Autodesk Inventor part; units mm, degrees
ref_plane "YZ Plane" through (0, 0, 0) normal (1, 0, 0) x (0, 1, 0)
ref_plane "XZ Plane" through (0, 0, 0) normal (0, 1, 0) x (-1, 0, 0)
ref_plane "XY Plane" through (0, 0, 0) normal (0, 0, 1) x (1, 0, 0)
sketch "Эскиз1" plane through (0, 0, 0) normal (0, 1, 0) x (-1, 0, 0)
  line L0 (7.1, -15.85) -> (-7.1, -15.85)
  line L1 (-7.1, -15.85) -> (-7.1, 15.85)
  line L2 (-7.1, 15.85) -> (7.1, 15.85)
  line L3 (7.1, 15.85) -> (7.1, -15.85)
  line L4 (7.1, -15.85) -> (-7.1, 15.85) construction
  line L5 (-7.1, -15.85) -> (7.1, 15.85) construction
  line L6 (9.1, -17.85) -> (-9.1, -17.85)
  line L7 (-9.1, -17.85) -> (-9.1, 17.85)
  line L8 (-9.1, 17.85) -> (9.1, 17.85)
  line L9 (9.1, 17.85) -> (9.1, -17.85)
  point P0 (0, 0)
  dimension "d0" = 14.2
  dimension "d1" = 31.7
  dimension "d2" = 2
extrude "Выдавливание1" add sketch "Эскиз1" along normal blind 7
sketch "Эскиз2" plane through (0, 7, 0) normal (0, 1, 0) x (1, 0, 0)
  line L0 (-9.1, 17.85) -> (-9.1, -17.85)
  line L1 (-9.1, -17.85) -> (9.1, -17.85)
  line L2 (9.1, -17.85) -> (9.1, 17.85)
  line L3 (9.1, 17.85) -> (-9.1, 17.85)
  point P0 (0, 0)
extrude "Выдавливание2" add sketch "Эскиз2" along normal blind 3
sketch "Эскиз4" plane through (9.1, 0, -17.85) normal (0, 0, -1) x (-1, 0, 0)
  line L0 (0, 0) -> (0, 10) construction
  line L1 (0, 0) -> (0, 10) construction
  line L2 (0, 0) -> (18.2, 0) construction
  line L3 (18.2, 0) -> (18.2, 10) construction
  line L4 (18.2, 0) -> (18.2, 10) construction
  line L5 (0, 0) -> (0, 10)
  line L6 (0, 0) -> (0, 10)
  line L7 (18.2, 0) -> (0, 0)
  line L8 (0, 0) -> (18.2, 0)
  line L9 (18.2, 0) -> (18.2, 10)
  line L10 (5.972, 10) -> (0, 10)
  line L11 (0, 10) -> (18.2, 10)
  line L12 (0, 0) -> (0, 10)
  line L13 (0, 10) -> (0, 7)
  line L14 (2, 0) -> (2, 7)
  line L15 (2, 7) -> (16.2, 7)
  line L16 (16.2, 7) -> (16.2, 0)
  point P0 (9.1, 0)
  point P1 (18.2, 7)
  point P2 (0, 5)
  point P3 (18.2, 5)
  point P4 (16.2, 0)
  dimension "d1" = 31.7
  dimension "d15" = 2
  dimension "d16" = 2
extrude "Выдавливание4" cut sketch "Эскиз4" against normal blind 3 contours L14 L15 L16 L7
sketch "Эскиз5" plane through (0, 10, 0) normal (0, 1, 0) x (1, 0, 0)
  line L0 (0, 0) -> (0, -28.4562) construction
  circle A0 centre (0, -22.85) radius 1.6
  circle A1 centre (0, 22.85) radius 1.6
  line L1 (-9.1, -17.85) -> (9.1, -17.85)
  line L2 (9.1, 17.85) -> (-9.1, 17.85)
  arc A2 (2.6208, 25.1698) -> (-2.6208, 25.1698) centre (0, 22.85) ccw
  arc A3 (-2.6208, -25.1698) -> (2.6208, -25.1698) centre (0, -22.85) ccw
  line L3 (9.1, 17.85) -> (7.1, 17.85)
  line L4 (9.1, 17.85) -> (2.6208, 25.1698)
  line L5 (-9.1, 17.85) -> (-2.6208, 25.1698)
  line L6 (-9.1, -17.85) -> (-2.6208, -25.1698)
  line L7 (9.1, -17.85) -> (9.1, 17.85)
  line L8 (9.1, -17.85) -> (2.6208, -25.1698)
  dimension "d32" = 3.2
  dimension "d33" = 3.2
  dimension "d34" = 5
  dimension "d35" = 5
  dimension "d36" = 7
  dimension "d37" = 7
extrude "Выдавливание5" add sketch "Эскиз5" against normal blind 3
sketch "Эскиз6" plane through (0, 7, 0) normal (0, -1, 0) x (1, 0, 0)
  circle A0 centre (0, -8.65) radius 1.5 construction
  circle A1 centre (0, -8.65) radius 1.6
  point P0 (0, 0)
  dimension "d38" = 3.2
extrude "Выдавливание6" cut sketch "Эскиз6" against normal blind 10
chamfer "Фаска1" distance 1.65 angle 45 1 edges at (-1.6, 10, -8.65)
properties part number "креп_опт" material "Полипропилен"
Model file for the job. Use its own axes, mm. A direction names the side the tool comes from. Give positions to 0.01 mm unless a question says otherwise; leave off trailing zeros. Order: outer loops, then holes, each group sorted by start corner. A loop starts at its lowest first (then second) coordinate and runs counter-clockwise, first axis right, second up.
1) Saw through at D-D, the plane x = -4.25. Write the cut outline in (y, z).
2) Saw through at C-C, the plane y = 1.25. Write the cut outline in (x, z), then the cut area to 3 significant figures.
3) Saw through at A-A, the plane z = -8.65. Write the cut outline in (x, y), then the cut area to 3 significant figures.
4) Wall check: probe 1 along Z at (x, y) = (0, 7.85); probe 2 along Z at (x, y) = (0, 9.3); probe 3 along X at (y, z) = (5.25, 2). Give the ranges that are in metal, low to high.
5) Saw through at B-B, the plane y = 7.5. Write the cut outline in (x, z), then the cut area to 3 significant figures.
6) Mould opens along Z. For faces 1 (the flat face through (5.906, 8.521, -21.459)), 2 (the cylindrical face through (-0.35, 8.52, 24.41)), 3 (the flat face through (7.1, 3, -1)) say: +Z half, -Z half, draft (parallel to the pull), parting line (faces both ways), or undercut.
7) 3-axis set-ups, long thin cutter, end or side, ignore diameter. For faces 4 (the flat face through (0, 7, 21)), 5 (the flat face through (0, 3, 15.85)), 6 (the flat face through (-9.1, 5, 0)), 7 (the flat face through (7.5, 0, 4)), 8 (the flat face through (8, 3, -17.85)): which of +Z, -Z, +X, -X, +Y, -Y reach the whole face in a straight line?
8) Pin check, flat tips, straight feed: pin 1 (4 mm diameter, centred on x = 0, z = -22.85, fed in from -Y); pin 2 (2 mm diameter, centred on x = 8.5, y = 2.5, fed in from -Z); pin 3 (1.5 mm diameter, centred on x = -1.5, y = 3, fed in from +Z). Stop position of each tip, or through.
Computed:
1. outline: (0, 15.85) - (7, 15.85) - (7, -23.33) - (10, -23.33) - (10, 23.33) - (7, 23.33) - (7, 17.85) - (0, 17.85) - close
2. outline: (-9.1, -17.85) - (-7.1, -17.85) - (-7.1, 15.85) - (7.1, 15.85) - (7.1, -17.85) - (9.1, -17.85) - (9.1, 17.85) - (-9.1, 17.85) - close
2. area: 171 mm2
3. outline: (-9.1, 0) - (-7.1, 0) - (-7.1, 7) - (-1.6, 7) - (-1.6, 8.35) - (-3.25, 10) - (-9.1, 10) - close; (1.6, 7) - (7.1, 7) - (7.1, 0) - (9.1, 0) - (9.1, 10) - (3.25, 10) - (1.6, 8.35) - close
3. area: 70.3 mm2
4. probe 1: z = -26.35 to -24.45, -21.25 to -10.25, -7.05 to 21.25, 24.45 to 26.35
4. probe 2: z = -26.35 to -24.45, -21.25 to -11.2, -6.1 to 21.25, 24.45 to 26.35
4. probe 3: x = -9.1 to -7.1, 7.1 to 9.1
5. outline: (-9.1, -17.85) - (-2.62, -25.17) arc R3.5 ccw to (2.62, -25.17) - (9.1, -17.85) - (9.1, 17.85) - (2.62, 25.17) arc R3.5 ccw to (-2.62, 25.17) - (-9.1, 17.85) - close; hole circle Ø3.2 at (0, -22.85); hole circle Ø3.2 at (0, -8.65); hole circle Ø3.2 at (0, 22.85)
5. area: 806 mm2
6. face 1: -Z half
6. face 2: undercut
6. face 3: draft
7. face 4: +Z, +X, -X, -Y
7. face 5: -Z, -Y
7. face 6: +Z, -Z, -X, +Y, -Y
7. face 7: +Z, -Z, +X, -X, -Y
7. face 8: -Z, +X, -X, -Y
8. pin 1: stops at y = 7
8. pin 2: stops at z = -17.85
8. pin 3: stops at z = 17.85
